Part model, mm, in its own coordinate system. Face numbers are marked on the shaded views. A direction names the side the tool comes from. Round coordinates to 2 decimals unless told otherwise and drop trailing zeros. Write each loop counter-clockwise with the first axis right and the second up, starting at its lowest first coordinate (ties: lowest second). Pieces come first, ordered by that corner, then holes. Notation, with made-up numbers: M -30,5 L -4,5 A26 ccw -4,35 Z; hole C 52.5,85 d7. An arc over 180 degrees is marked long. Use a Markdown table: item, result. Add a question column.
1) Slice it at D-D on x = 2. Write the cut outline in (y, z).
2) Slice it at C-C on z = 0. Give the number of separate pieces and of enclosed holes in the cut face, plus the area to 3 significant figures.
3) Which spindle directions (+Z, -Z, +X, -X, +Y, -Y) get a long thin tool onto all of the face, cutting with end or side? Do the marked faces 4, 5 and 6. Say none if no direction does.
4) Drop flat-ended pins along their axis: P1, Ø5, axis at x = 16.5, y = 25, coming from the -Z side; P2, Ø5, axis at x = 30, y = 31.5, coming from the +Z side; P3, Ø13, axis at y = 0, z = 0, coming from the +X side; P4, Ø8.5, axis at x = 23, z = -3, coming from the +Y side. Give the stop position or say it passes through.
5) Wall check: probe 1 along Y at (x, z) = (14.1, 0); probe 2 along Y at (x, z) = (27, 8); probe 3 along Z at (x, y) = (22, 32.75). Give the ranges that are in metal, low to high.
6) Two-plate mould, pull along Y, no slides. Class the marked faces 1, 2 and 3: released by +Y, released by -Y, zero draft, split by the parting line, or undercut.
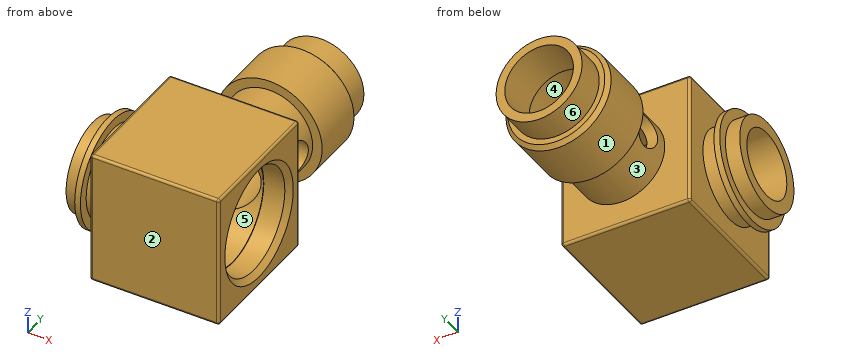
```python
from build123d import *

# Parameters (mm, degrees)
SKETCH_2_R           = 9
EXTRUDE_1_DEPTH      = 25
SKETCH_3_R           = 11
EXTRUDE_2_DEPTH      = 12
SKETCH_4_R           = 9
EXTRUDE_3_DEPTH      = 6
SKETCH_5_R           = 10.75
CUT_EXTRUDE_1_DEPTH  = 23.1
CUT_EXTRUDE_START    = -8.5
SKETCH_6_R           = 8.5
CUT_EXTRUDE_2_DEPTH  = 7
CUT_EXTRUDE_3_REACH  = 43.5
SKETCH_8_R           = 6.75
SKETCH_9_R           = 3.5
CUT_EXTRUDE_4_DEPTH  = 35.7000001
SKETCH_10_R          = 10.75
EXTRUDE_4_DEPTH      = 5.95
CHAMFER_1_SIZE       = 0.828
SKETCH_12_W          = 28
SKETCH_12_H          = 28
SKETCH_12_R          = 13
EXTRUDE_5_DEPTH      = 27
CUT_EXTRUDE_5_REACH  = 30
SKETCH_13_R          = 6.75
CUT_EXTRUDE_6_REACH  = 59
SKETCH_14_R          = 7.172
SKETCH_16_R          = 10.8985
CUT_EXTRUDE_7_DEPTH  = 5.5
CHAMFER_3_SIZE       = 1.1015
CUT_EXTRUDE_11_REACH = 7.95
SKETCH_18_R          = 10.75
FILLET_1_R           = 0.5


with BuildPart() as part:
    # Эскиз1 → Повернуть1 (revolve)
    with BuildSketch(Plane.XY):
        Polygon((0, -7), (11.6, -7), (11.6, 0), (34.7, 0), (34.7, -10.5), (34.7, -14), (7.7, -14), (7.7, -9.5), (4.2, -9.5), (4.2, -11.5), (3, -11.5), (3, -9.5), (0, -9.5), align=None)
    revolve(axis=Axis((0, 0, 0), (1, 0, 0)))

    # Эскиз2 → Бобышка-Вытянуть1 (add)
    with BuildSketch(Plane(origin=(0, 0, 0), x_dir=(1, 0, 0), z_dir=(0, 1, 0))):
        with Locations((22, 0)):
            Circle(SKETCH_2_R)
    extrude(amount=EXTRUDE_1_DEPTH)

    # Эскиз3 → Бобышка-Вытянуть2 (add)
    with BuildSketch(Plane(origin=(0, 25, 0), x_dir=(1, 0, 0), z_dir=(0, 1, 0))):
        with Locations((22, 0)):
            Circle(SKETCH_3_R)
    extrude(amount=EXTRUDE_2_DEPTH)

    # Эскиз4 → Бобышка-Вытянуть3 (add)
    with BuildSketch(Plane(origin=(0, 37, 0), x_dir=(1, 0, 0), z_dir=(0, 1, 0))):
        with Locations((22, 0)):
            Circle(SKETCH_4_R)
    extrude(amount=EXTRUDE_3_DEPTH)

    # Эскиз5 → Вырез-Вытянуть1 (cut)
    with BuildSketch(Plane(origin=(34.7, 0, 0), x_dir=(0, 0, -1), z_dir=(1, 0, 0))):
        Circle(SKETCH_5_R)
    extrude(amount=-CUT_EXTRUDE_1_DEPTH, mode=Mode.SUBTRACT)

    # Эскиз6 → Вырез-Вытянуть2 (cut)
    with BuildSketch(Plane(origin=(0, 43, 0), x_dir=(1, 0, 0), z_dir=(0, 1, 0)).offset(CUT_EXTRUDE_START)):
        with Locations((22, 0)):
            Circle(SKETCH_6_R)
    extrude(amount=-CUT_EXTRUDE_2_DEPTH, mode=Mode.SUBTRACT)

    # Эскиз8 → Вырез-Вытянуть3 (cut, up to next)
    with BuildSketch(Plane(origin=(0, 27.5, 0), x_dir=(1, 0, 0), z_dir=(0, 1, 0)), mode=Mode.PRIVATE) as cut_extrude_3_sk1:
        with Locations((22, 0)):
            Circle(SKETCH_8_R)
    cut_extrude_3_tool1 = extrude(cut_extrude_3_sk1.sketch, amount=-CUT_EXTRUDE_3_REACH, mode=Mode.PRIVATE) & part.part
    add(cut_extrude_3_tool1.solids().sort_by_distance((22, 27.5, 0))[0], mode=Mode.SUBTRACT)

    # Эскиз9 → Вырез-Вытянуть4 (cut, through all)
    with BuildSketch(Plane(origin=(0, 0, 0), x_dir=(0, 0, -1), z_dir=(1, 0, 0))):
        with Locations((0, 20)):
            Circle(SKETCH_9_R)
    extrude(amount=CUT_EXTRUDE_4_DEPTH, mode=Mode.SUBTRACT)

    # Эскиз10 → Бобышка-Вытянуть4 (add)
    with BuildSketch(Plane(origin=(34.7, 0, 0), x_dir=(0, 0, -1), z_dir=(1, 0, 0))):
        Circle(SKETCH_10_R)
    extrude(amount=-EXTRUDE_4_DEPTH)

    # Фаска1
    chamfer_1_edges = [part.edges().sort_by_distance(p)[0] for p in [
        (11, 37, 0),
    ]]
    chamfer(chamfer_1_edges, length=CHAMFER_1_SIZE)

    # Эскиз12 → Бобышка-Вытянуть5 (add)
    with BuildSketch(Plane(origin=(34.7, 0, 0), x_dir=(0, 0, -1), z_dir=(1, 0, 0))):
        Rectangle(SKETCH_12_W, SKETCH_12_H)
        Circle(SKETCH_12_R, mode=Mode.SUBTRACT)
    extrude(amount=-EXTRUDE_5_DEPTH)

    # Эскиз13 → Вырез-Вытянуть5 (cut, up to next)
    with BuildSketch(Plane(origin=(0, 14, 0), x_dir=(1, 0, 0), z_dir=(0, 1, 0)), mode=Mode.PRIVATE) as cut_extrude_5_sk1:
        with Locations((22, 0)):
            Circle(SKETCH_13_R)
    cut_extrude_5_tool1 = extrude(cut_extrude_5_sk1.sketch, amount=-CUT_EXTRUDE_5_REACH, mode=Mode.PRIVATE) & part.part
    add(cut_extrude_5_tool1.solids().sort_by_distance((22, 14, 0))[0], mode=Mode.SUBTRACT)

    # Эскиз14 → Вырез-Вытянуть6 (cut, up to next)
    with BuildSketch(Plane(origin=(0, 43, 0), x_dir=(1, 0, 0), z_dir=(0, 1, 0)), mode=Mode.PRIVATE) as cut_extrude_6_sk1:
        with Locations((22, 0)):
            Circle(SKETCH_14_R)
    cut_extrude_6_tool1 = extrude(cut_extrude_6_sk1.sketch, amount=-CUT_EXTRUDE_6_REACH, mode=Mode.PRIVATE) & part.part
    add(cut_extrude_6_tool1.solids().sort_by_distance((22, 43, 0))[0], mode=Mode.SUBTRACT)

    # Эскиз16 → Вырез-Вытянуть7 (cut)
    with BuildSketch(Plane(origin=(34.7, 0, 0), x_dir=(0, 0, -1), z_dir=(1, 0, 0))):
        Circle(SKETCH_16_R)
    extrude(amount=-CUT_EXTRUDE_7_DEPTH, mode=Mode.SUBTRACT)

    # Фаска3
    chamfer_3_edges = [part.edges().sort_by_distance(p)[0] for p in [
        (34.7, 0, 10.8985),
    ]]
    chamfer(chamfer_3_edges, length=CHAMFER_3_SIZE)

    # Эскиз18 → Вырез-Вытянуть11 (cut, up to next)
    with BuildSketch(Plane.ZY.offset(-28.75), mode=Mode.PRIVATE) as cut_extrude_11_sk1:
        Circle(SKETCH_18_R)
    cut_extrude_11_tool1 = extrude(cut_extrude_11_sk1.sketch, amount=-CUT_EXTRUDE_11_REACH, mode=Mode.PRIVATE) & part.part
    add(cut_extrude_11_tool1.solids().sort_by_distance((28.75, 0, 0))[0], mode=Mode.SUBTRACT)

    # Скругление1
    fillet_1_edges = [part.edges().sort_by_distance(p)[0] for p in [
        (34.7, 0, 14),
        (34.7, -14, 0),
        (34.7, 0, -14),
        (34.7, 14, 0),
        (7.7, 0, -14),
        (21.2, 14, -14),
        (7.7, -14, 0),
        (21.2, -14, -14),
        (7.7, 0, 14),
        (21.2, -14, 14),
        (7.7, 14, 0),
        (21.2, 14, 14),
    ]]
    fillet(fillet_1_edges, radius=FILLET_1_R)


solid = part.part
```
Entries:
| question | item | result |
|---|---|---|
| 1 | outline | C 0,0 d19; hole C 0,0 d14 |
| 2 | separate pieces | 5 |
| 2 | enclosed holes | 0 |
| 2 | area | 316 mm^2 |
| 3 | face 4 | none |
| 3 | face 5 | +X |
| 3 | face 6 | +Y |
| 4 | P1 | stops at z = -10.58 |
| 4 | P2 | stops at z = 9.53 |
| 4 | P3 | passes through |
| 4 | P4 | stops at y = 43 |
| 5 | probe 1 | y = -14 to -10.75, 10.75 to 16.5, 23.5 to 27.5, 34.5 to 43 |
| 5 | probe 2 | y = -14 to -7.18, 7.18 to 14, 25 to 37 |
| 5 | probe 3 | z = -11 to -8.5, 8.5 to 11 |
| 6 | face 1 | zero draft |
| 6 | face 2 | released by -Y |
| 6 | face 3 | undercut |
